from build123d import *

# Parameters (mm, degrees)
SKETCH5_R          = 6.35
CUT_EXTRUDE1_DEPTH = 33.380549717
SKETCH7_W          = 25.4
SKETCH7_H          = 25.4
CUT_EXTRUDE2_DEPTH = 1
SKETCH8_R          = 0.8
CUT_EXTRUDE3_DEPTH = 33.380549717
SKETCH9_R          = 0.5
CUT_EXTRUDE4_DEPTH = 33.380549875


# Read off the part's stored shape, not the designer's step: Loft1
with BuildPart() as part:
    # Loft1 outline → Loft1 (revolve)
    with BuildSketch(Plane.XY):
        Polygon((0, 0), (17.96, 0), (22.5, 6), (0, 6), align=None)
    revolve(axis=Axis((0, 0, 0), (0, 1, 0)))

    # Sketch5 → Cut-Extrude1 (cut, through all)
    with BuildSketch(Plane(origin=(0, 6, 0), x_dir=(1, 0, 0), z_dir=(0, 1, 0))):
        with Locations(Location((0, 0, 0), (0, 0, 270))):
            Circle(SKETCH5_R)
    extrude(amount=-CUT_EXTRUDE1_DEPTH, mode=Mode.SUBTRACT)

    # Sketch7 → Cut-Extrude2 (cut)
    with BuildSketch(Plane(origin=(0, 6, 0), x_dir=(1, 0, 0), z_dir=(0, 1, 0))):
        Rectangle(SKETCH7_W, SKETCH7_H)
    extrude(amount=-CUT_EXTRUDE2_DEPTH, mode=Mode.SUBTRACT)

    # Sketch8 → Cut-Extrude3 (cut, through all)
    with BuildSketch(Plane.XY):
        with Locations((0, 4)):
            Circle(SKETCH8_R)
    extrude(amount=-CUT_EXTRUDE3_DEPTH, mode=Mode.SUBTRACT)

    # Sketch9 → Cut-Extrude4 (cut, through all)
    with BuildSketch(Plane(origin=(0, 0, 0), x_dir=(0, 0, -1), z_dir=(1, 0, 0))):
        with Locations((0, 4)):
            Circle(SKETCH9_R)
    extrude(amount=-CUT_EXTRUDE4_DEPTH, mode=Mode.SUBTRACT)


solid = part.part
Could you check a few things on this model? Use its own coordinates, in mm. A direction names the side the tool comes from. Give positions to 0.01 mm unless a question says otherwise; leave off trailing zeros. Order: outer loops, then holes, each group sorted by start corner. A loop starts at its lowest first (then second) coordinate and runs counter-clockwise, first axis right, second up. Notation, with made-up numbers: (-22.75, 65) -> (31.25, 65) arc R20 cw to (31.25, 76) -> close; hole circle Ø7 at (60, 32.25). An arc over 180 degrees is marked (long way). Return JSON: item names as keys, results as strings.
1. For pin 1 Ø0.5 at (y, z) = (5.5, 5.5) entering from -X; pin 2 Ø3 at (y, z) = (5.5, -3) entering from +X; pin 3 Ø1.4 at (x, y) = (0, 4) entering from +Z; pin 4 Ø12 at (x, z) = (15, 13) entering from -Y, each with a flat end and sliding along its axis, tell me the tip position at first contact or that it passes through.
Answer list:
{"pin 1": "stops at x = -21.63", "pin 2": "stops at x = 22.44", "pin 3": "stops at z = 21.52", "pin 4": "stops at y = 0"}
2. I need wall thicknesses on line 1 (Y direction, x = -15, z = 0); line 2 (Y direction, x = 0, z = -10); line 3 (Y direction, x = -10.5, z = -8.5). Which ranges of each line are inside material? Lowest first, please. Write a range as from..to.
Answer list:
{"line 1": "y = 0..3.5, 4.5..6", "line 2": "y = 0..3.2, 4.8..5", "line 3": "y = 0..5"}
3. Imagine slicing it at A-A on x = 0. List the corners of the cut face in (y, z) for me.
Answer list:
{"outline": "(0, -17.96) -> (3.2, -20.38) -> (3.2, -6.35) -> (0, -6.35) -> close; (0, 6.35) -> (5, 6.35) -> (5, 12.7) -> (6, 12.7) -> (6, 22.5) -> (0, 17.96) -> close; (4.8, -21.59) -> (6, -22.5) -> (6, -12.7) -> (5, -12.7) -> (5, -6.35) -> (4.8, -6.35) -> close"}
4. On a 3-axis mill with a long thin cutter (end or side, diameter ignored), from which of +Z, -Z, +X, -X, +Y, -Y can I reach the whole of each face in a straight line? I mean faces 1 (the flat face through (-0.2, 5.5, 12.7)), 2 (the flat face through (0, 6, 15)), 3 (the cylindrical face through (-13.742, 4.496, 0.065)). Say none if no direction works.
Answer list:
{"face 1": "+Y", "face 2": "+Z, -Z, +X, -X, +Y", "face 3": "-X"}
5. Thinking about a two-plate mould opening in Z: for faces 4 (the flat face through (-3, 5, -6)), 5 (the cylindrical face through (0.43, 4.675, -13.839)), 6 (the conical face through (-3.955, 0.375, 17.81)), which applies, pulls with the +Z half, pulls with the -Z half, needs draft (parallel to the pull), parting line crosses it, or undercut?
Answer list:
{"face 4": "undercut", "face 5": "needs draft", "face 6": "parting line crosses it"}
